Autodesk Inventor part; units mm, degrees
ref_plane "YZ Plane" through (0, 0, 0) normal (1, 0, 0) x (0, 1, 0)
ref_plane "XZ Plane" through (0, 0, 0) normal (0, 1, 0) x (-1, 0, 0)
ref_plane "XY Plane" through (0, 0, 0) normal (0, 0, 1) x (1, 0, 0)
sketch "Sketch1" plane through (0, 0, 0) normal (0, 0, 1) x (1, 0, 0)
  arc A0 (7.6035, 1.5) -> (7.6035, -1.5) centre (0, 0) ccw
  arc A1 (47.3965, -1.5) -> (47.3965, 1.5) centre (55, 0) ccw
  line L0 (-11, -11) -> (66, -11)
  line L1 (66, -11) -> (66, 11)
  line L2 (66, 11) -> (42, 11)
  line L3 (42, 11) -> (42, 1.5)
  line L4 (42, 1.5) -> (47.3965, 1.5)
  line L5 (13, 11) -> (-11, 11)
  line L6 (-11, 11) -> (-11, -11)
  line L7 (13, 11) -> (13, 1.5)
  line L8 (13, 1.5) -> (7.6035, 1.5)
  line L9 (7.6035, -1.5) -> (13, -1.5)
  line L10 (13, -1.5) -> (13, -5)
  line L11 (13, -5) -> (42, -5)
  line L12 (42, -5) -> (42, -1.5)
  line L13 (42, -1.5) -> (47.3965, -1.5)
  dimension "d0" = 15.5
  dimension "d1" = 55
  dimension "d2" = 11
  dimension "d3" = 11
  dimension "d4" = 11
  dimension "d7" = 1.5
  dimension "d8" = 1.5
  dimension "d9" = 13
  dimension "d10" = 13
  dimension "d11" = 6
extrude "Extrusion1" add sketch "Sketch1" along normal blind 58
chamfer "Chamfer1" distance 5 angle 45 6 edges at (-11, 11, 29) (-11, -11, 29) (66, 11, 29) (66, -11, 29) (42, 11, 29) (13, 11, 29)
chamfer "Chamfer2" distance 3.5 angle 45 2 edges at (42, -5, 29) (13, -5, 29)
sketch "Sketch2" plane through (16.5, -5, 0) normal (0, 1, 0) x (1, 0, 0)
  line L0 (22, 0) -> (22, -58)
  line L1 (22, 0) -> (0, 0)
  circle A0 centre (16, -20) radius 4
  circle A1 centre (16, -38) radius 4
  point P0 (-16.5, 0)
  dimension "d20" = 8
  dimension "d21" = 6
  dimension "d22" = 20
  dimension "d23" = 18
extrude "Extrusion2" cut sketch "Sketch2" against normal up to next
properties part number "ChimeraXCarriageLowTest"
Could you check a few things on this model? Use its own coordinates, in mm. A direction names the side the tool comes from. Coordinates: 2 decimals unless noted, no trailing zeros. Write each loop counter-clockwise with the first axis right and the second up, starting at its lowest first coordinate (ties: lowest second). Pieces come first, ordered by that corner, then holes. Notation, with made-up numbers: (53.5, 32) - (64.5, 32) arc R13 ccw to (64.5, 56) - close; hole circle Ø1 at (52, 84.5). An arc over 180 degrees is marked (long way). Put each result on its own line as item: value. Start each with the question number.
Q1. Please list where these lines run through material, in increasing order: L1, parallel to Z at x = 32.5, y = -7.75; L2, parallel to X at y = 0, z = 41; L3, parallel to X at y = 4, z = 40.
Q2. I'm going to push flat-ended pins straight in: P1, Ø12, axis at x = 24, y = -6.5, coming from the -Z side; P2, Ø1, axis at x = 48.5, y = -1.5, coming from the +Z side; P3, Ø2.5, axis at x = 45, z = 33.5, coming from the +Y side; P4, Ø11, axis at x = 29, z = 40.5, coming from the +Y side. Where does each tip first touch, or does it pass through?
Q3. Thinking about a two-plate mould opening in Y: for faces 4 (the flat face through (45, 9, 29)), 5 (the flat face through (45, 1.5, 29)), 6 (the flat face through (27, -11, 29)), which applies, pulls with the +Y half, pulls with the -Y half, needs draft (parallel to the pull), parting line crosses it, or undercut?
Q4. I want a section at A-A on x = 32.5. Write out the boundary of the cut face in (y, z).
Q5. I want a section at D-D on x = 55. Write out the boundary of the cut face in (y, z).
Q6. Which directions (+Z, -Z, +X, -X, +Y, -Y) give clear straight access to the entire face, cutting with the end or side of a thin tool? Please do faces 1 (the cylindrical face through (29.55, -7.96, 17.3)), 2 (the flat face through (42, 4, 29)), 3 (the flat face through (10, 1.5, 29)).
Q7. I want a section at C-C on y = 0. Write out the boundary of the cut face in (x, z), plus the area to 3 significant figures.
Checks:
1. L1: 0 to 16, 24 to 34, 42 to 58
1. L2: -11 to -7.75, 62.75 to 66
1. L3: -11 to -6.64, 6.64 to 13, 42 to 48.36, 61.64 to 66
2. P1: z = 0
2. P2: through
2. P3: y = 10.25
2. P4: y = -5
3. face 4: pulls with the +Y half
3. face 5: undercut
3. face 6: pulls with the -Y half
4. outline: (-11, 0) - (-5, 0) - (-5, 16) - (-11, 16) - close; (-11, 24) - (-5, 24) - (-5, 34) - (-11, 34) - close; (-11, 42) - (-5, 42) - (-5, 58) - (-11, 58) - close
5. outline: (-11, 0) - (-7.75, 0) - (-7.75, 58) - (-11, 58) - close; (7.75, 0) - (11, 0) - (11, 58) - (7.75, 58) - close
6. face 1: +Y, -Y
6. face 2: +Z, -Z, +Y
6. face 3: +Z, -Z
7. outline: (-11, 0) - (-7.75, 0) - (-7.75, 58) - (-11, 58) - close; (62.75, 0) - (66, 0) - (66, 58) - (62.75, 58) - close
7. area: 377 mm²
